Check sheet for the modelled part. Datum: model origin and axes. Units: mm. Face numbers are marked on the shaded views. A direction names the side the tool comes from. Give positions to 0.01 mm unless a question says otherwise; leave off trailing zeros. Write each loop counter-clockwise with the first axis right and the second up, starting at its lowest first coordinate (ties: lowest second). Pieces come first, ordered by that corner, then holes. Notation, with made-up numbers: (31, 59) -> (74, 59) arc R20 ccw to (74, 70) -> close; hole circle Ø1 at (67.25, 6). An arc over 180 degrees is marked (long way). Return JSON: item names as keys, results as strings.
from build123d import *

# Parameters (mm, degrees)
SKETCH1_R           = 19.05
SKETCH1_R_2         = 2.5796875
SKETCH1_W           = 6.35
SKETCH1_H           = 6.35
BOSS_EXTRUDE1_DEPTH = 6.35


with BuildPart() as part:
    # Sketch1 → Boss-Extrude1 (new body)
    with BuildSketch(Plane(origin=(0, 0, 0), x_dir=(1, 0, 0), z_dir=(0, 1, 0))):
        Circle(SKETCH1_R)
        with Locations((0, 12.7)):
            Circle(SKETCH1_R_2, mode=Mode.SUBTRACT)
        with Locations((10.998522628, -6.35)):
            Circle(SKETCH1_R_2, mode=Mode.SUBTRACT)
        with Locations((-10.998522628, -6.35)):
            Circle(SKETCH1_R_2, mode=Mode.SUBTRACT)
        Rectangle(SKETCH1_W, SKETCH1_H, mode=Mode.SUBTRACT)
        with BuildLine():
            ThreePointArc((1.190625, -10.903378281), (0, -9.712753281), (-1.190625, -10.903378281))
            ThreePointArc((-1.190625, -10.903378281), (0, -12.094003281), (1.190625, -10.903378281))
        make_face(mode=Mode.SUBTRACT)
    extrude(amount=BOSS_EXTRUDE1_DEPTH)


solid = part.part
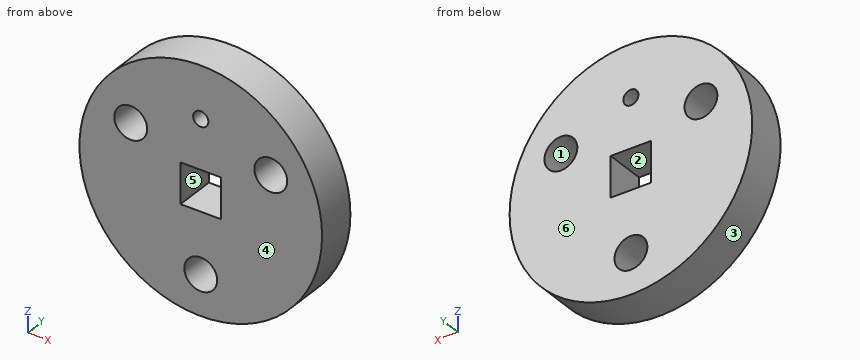
(1) Depth check by flat-ended pin: pin 1 Ø4 at (x, z) = (-11, 6.35) entering from -Y; pin 2 Ø3 at (x, y) = (7, 2) entering from -Z; pin 3 Ø3 at (x, y) = (0.5, 4.5) entering from -Z; pin 4 Ø3 at (x, y) = (-12.5, 2) entering from +Z. Enter the tip coordinate at first touch or a pass-through.
Reply:
{"pin 1": "through", "pin 2": "z = -18.24", "pin 3": "z = -19.05", "pin 4": "z = 15.55"}
(2) Release check for a two-part mould opening along Z. For the marked faces 1, 2, 3 and 4 record: pulls with the +Z half, pulls with the -Z half, needs draft (parallel to the pull), parting line crosses it, or undercut.
Reply:
{"face 1": "undercut", "face 2": "undercut", "face 3": "parting line crosses it", "face 4": "needs draft"}
(3) Cross-section at D-D on z = 5.5. Enter the section's corners in (x, y), then the cut area to 3 significant figures.
Reply:
{"outline": "(-18.24, 0) -> (-13.43, 0) -> (-13.43, 6.35) -> (-18.24, 6.35) -> close; (-8.56, 0) -> (8.56, 0) -> (8.56, 6.35) -> (-8.56, 6.35) -> close; (13.43, 0) -> (18.24, 0) -> (18.24, 6.35) -> (13.43, 6.35) -> close", "area": "170 mm^2"}
(4) Cross-section at A-A on x = 0. Enter the section's corners in (y, z) (3 decimals).
Reply:
{"outline": "(0, -19.05) -> (6.35, -19.05) -> (6.35, -15.28) -> (0, -15.28) -> close; (0, -10.12) -> (6.35, -10.12) -> (6.35, -3.175) -> (0, -3.175) -> close; (0, 3.175) -> (6.35, 3.175) -> (6.35, 9.713) -> (0, 9.713) -> close; (0, 12.094) -> (6.35, 12.094) -> (6.35, 19.05) -> (0, 19.05) -> close"}
(5) Cross-section at B-B on z = 0. Enter the section's corners in (x, y) (3 decimals), then the cut area to 3 significant figures.
Reply:
{"outline": "(-19.05, 0) -> (-3.175, 0) -> (-3.175, 6.35) -> (-19.05, 6.35) -> close; (3.175, 0) -> (19.05, 0) -> (19.05, 6.35) -> (3.175, 6.35) -> close", "area": "202 mm^2"}
(6) Thickness scan on L1, parallel to Z at x = 0, y = 4.5 (3 decimals); L2, parallel to X at y = 3, z = 6.35; L3, parallel to Z at x = 0.5, y = 4 (3 decimals). Record the ranges inside material, lowest first.
Reply:
{"L1": "-19.05 to -15.28, -10.12 to -3.175, 3.175 to 9.713, 12.094 to 19.05", "L2": "-17.96 to -13.58, -8.42 to 8.42, 13.58 to 17.96", "L3": "-19.043 to -15.231, -10.169 to -3.175, 3.175 to 9.823, 11.984 to 19.043"}
(7) Cross-section at C-C on x = 12. Enter the section's corners in (y, z), then the cut area to 3 significant figures.
Reply:
{"outline": "(0, -14.8) -> (6.35, -14.8) -> (6.35, 3.97) -> (0, 3.97) -> close; (0, 8.73) -> (6.35, 8.73) -> (6.35, 14.8) -> (0, 14.8) -> close", "area": "158 mm^2"}
(8) Set-up check for the marked faces 5 and 6: record each of +Z, -Z, +X, -X, +Y, -Y from which the full face is reachable in a straight line by a thin tool's end or side.
Reply:
{"face 5": "+Y, -Y", "face 6": "+Z, -Z, +X, -X, +Y"}
